For this review, take the finished solid that the model builds, in its own axes (mm). Face numbers are marked on the shaded views. Round coordinates to 2 decimals unless told otherwise and drop trailing zeros. Order: outer loops, then holes, each group sorted by start corner. A loop starts at its lowest first (then second) coordinate and runs counter-clockwise, first axis right, second up. Notation, with made-up numbers: M -10,-11 L 6,-11 A11 cw 6,7 Z; hole C -3,2.25 d5. An arc over 180 degrees is marked long. Put each result on its own line as item: value.
from build123d import *

# Parameters (mm, degrees)
SKETCH1_R           = 1.7859375
SKETCH1_R_2         = 12.7
BOSS_EXTRUDE1_DEPTH = 3.175
SKETCH2_W           = 6.35
SKETCH2_H           = 38.1
BOSS_EXTRUDE2_DEPTH = 17.7165
SKETCH3_W           = 50.8
SKETCH3_H           = 38.1
SKETCH3_R           = 4.7625
BOSS_EXTRUDE3_DEPTH = 3.175
SKETCH4_W           = 6.35
SKETCH4_H           = 38.1
BOSS_EXTRUDE4_DEPTH = 6.35
FILLET1_R           = 2.54
CUT_EXTRUDE2_REACH  = 94.617
SKETCH6_R           = 1.7859375


with BuildPart() as part:
    # Sketch1 → Boss-Extrude1 (new body)
    with BuildSketch(Plane.XY):
        Polygon((25.4, -19.05), (25.4, 49.157882323), (61.857882323, 49.157882323), (61.857882323, 61.857882323), (19.05, 61.857882323), (-19.05, 61.857882323), (-61.857882323, 61.857882323), (-61.857882323, 49.157882323), (-25.4, 49.157882323), (-25.4, -19.05), (-25.4, -49.157882323), (-61.857882323, -49.157882323), (-61.857882323, -61.857882323), (-19.05, -61.857882323), (19.05, -61.857882323), (61.857882323, -61.857882323), (61.857882323, -49.157882323), (25.4, -49.157882323), align=None)
        with Locations((-55.507882323, -55.507882323)):
            Circle(SKETCH1_R, mode=Mode.SUBTRACT)
        with Locations((55.507882323, -55.507882323)):
            Circle(SKETCH1_R, mode=Mode.SUBTRACT)
        Circle(SKETCH1_R_2, mode=Mode.SUBTRACT)
        with Locations((-55.507882323, 55.507882323)):
            Circle(SKETCH1_R, mode=Mode.SUBTRACT)
        with Locations((55.507882323, 55.507882323)):
            Circle(SKETCH1_R, mode=Mode.SUBTRACT)
    extrude(amount=BOSS_EXTRUDE1_DEPTH)

    # Sketch2 → Boss-Extrude2 (add)
    with BuildSketch(Plane.XY.offset(3.175)):
        with Locations((22.225, 0)):
            Rectangle(SKETCH2_W, SKETCH2_H)
        with Locations((-22.225, 0)):
            Rectangle(SKETCH2_W, SKETCH2_H)
    extrude(amount=BOSS_EXTRUDE2_DEPTH)

    # Sketch3 → Boss-Extrude3 (add)
    with BuildSketch(Plane.XY.offset(20.8915)):
        Rectangle(SKETCH3_W, SKETCH3_H)
        Circle(SKETCH3_R, mode=Mode.SUBTRACT)
    extrude(amount=BOSS_EXTRUDE3_DEPTH)

    # Sketch4 → Boss-Extrude4 (add)
    with BuildSketch(Plane.XY.offset(24.0665)):
        with Locations((11.0236, 0)):
            Rectangle(SKETCH4_W, SKETCH4_H)
        with Locations((-11.0236, 0)):
            Rectangle(SKETCH4_W, SKETCH4_H)
    extrude(amount=BOSS_EXTRUDE4_DEPTH)

    # Fillet1
    fillet1_edges = [part.edges().sort_by_distance(p)[0] for p in [
        (61.857882323, -49.157882323, 1.5875),
        (61.857882323, -61.857882323, 1.5875),
        (-61.857882323, -61.857882323, 1.5875),
        (-61.857882323, -49.157882323, 1.5875),
        (-25.4, -49.157882323, 1.5875),
        (-25.4, 49.157882323, 1.5875),
        (-61.857882323, 49.157882323, 1.5875),
        (-61.857882323, 61.857882323, 1.5875),
        (61.857882323, 61.857882323, 1.5875),
        (61.857882323, 49.157882323, 1.5875),
        (25.4, 49.157882323, 1.5875),
        (25.4, -49.157882323, 1.5875),
    ]]
    fillet(fillet1_edges, radius=FILLET1_R)

    # Sketch6 → Cut-Extrude2 (cut, up to next)
    with BuildSketch(Plane(origin=(0, 0, 0), x_dir=(-1, 0, 0), z_dir=(0, 0, -1)), mode=Mode.PRIVATE) as cut_extrude2_sk1:
        with Locations((-22.225, -12.7)):
            Circle(SKETCH6_R)
    cut_extrude2_tool1 = extrude(cut_extrude2_sk1.sketch, amount=-CUT_EXTRUDE2_REACH, mode=Mode.PRIVATE) & part.part
    # Sketch6 → Cut-Extrude2 (cut, up to next)
    with BuildSketch(Plane(origin=(0, 0, 0), x_dir=(-1, 0, 0), z_dir=(0, 0, -1)), mode=Mode.PRIVATE) as cut_extrude2_sk2:
        with Locations((-22.225, 12.7)):
            Circle(SKETCH6_R)
    cut_extrude2_tool2 = extrude(cut_extrude2_sk2.sketch, amount=-CUT_EXTRUDE2_REACH, mode=Mode.PRIVATE) & part.part
    # Sketch6 → Cut-Extrude2 (cut, up to next)
    with BuildSketch(Plane(origin=(0, 0, 0), x_dir=(-1, 0, 0), z_dir=(0, 0, -1)), mode=Mode.PRIVATE) as cut_extrude2_sk3:
        with Locations((22.225, 12.7)):
            Circle(SKETCH6_R)
    cut_extrude2_tool3 = extrude(cut_extrude2_sk3.sketch, amount=-CUT_EXTRUDE2_REACH, mode=Mode.PRIVATE) & part.part
    # Sketch6 → Cut-Extrude2 (cut, up to next)
    with BuildSketch(Plane(origin=(0, 0, 0), x_dir=(-1, 0, 0), z_dir=(0, 0, -1)), mode=Mode.PRIVATE) as cut_extrude2_sk4:
        with Locations((22.225, -12.7)):
            Circle(SKETCH6_R)
    cut_extrude2_tool4 = extrude(cut_extrude2_sk4.sketch, amount=-CUT_EXTRUDE2_REACH, mode=Mode.PRIVATE) & part.part
    add(cut_extrude2_tool1.solids().sort_by_distance((22.225, -12.7, 0))[0], mode=Mode.SUBTRACT)
    add(cut_extrude2_tool2.solids().sort_by_distance((22.225, 12.7, 0))[0], mode=Mode.SUBTRACT)
    add(cut_extrude2_tool3.solids().sort_by_distance((-22.225, 12.7, 0))[0], mode=Mode.SUBTRACT)
    add(cut_extrude2_tool4.solids().sort_by_distance((-22.225, -12.7, 0))[0], mode=Mode.SUBTRACT)


solid = part.part
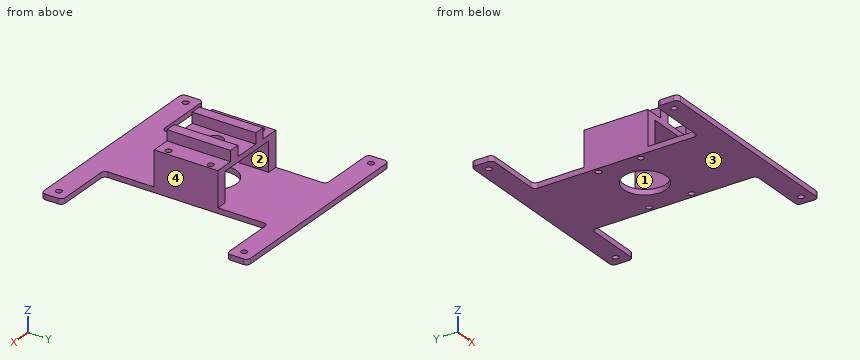
(1) Draft analysis for pull direction Z (two halves, no side actions). For the marked faces 1, 2, 3 and 4, state which applies: released by +Z, released by -Z, zero draft, split by the parting line, or undercut.
A:
face 1: undercut
face 2: undercut
face 3: released by -Z
face 4: zero draft
(2) To check wall thickness, follow L1, parallel to X at y = -8, z = 16; L2, parallel to Y at x = -6.5, z = 2; L3, parallel to Z at x = 13.5, y = -13 (1 decimal). State the ranges of each line that lie inside material, in increasing order.
A:
L1: x = -25.4 to -19.05, 19.05 to 25.4
L2: y = -61.86 to -10.91, 10.91 to 61.86
L3: z = 0 to 3.2, 20.9 to 30.4
(3) Insertion check: pin 1 Ø1.9 at (y, z) = (-6.5, 26.5) entering from -X; pin 2 Ø5.5 at (x, y) = (-17, -4.5) entering from +Z; pin 3 Ø5.5 at (x, y) = (-55.51, 55.51) entering from +Z (3 decimals); pin 4 Ø3 at (x, y) = (22.225, 12.7) entering from -Z. Each pin has a flat end and moves straight along its axis. Give the tip position at first contact, or say it passes through.
A:
pin 1: stops at x = -14.2
pin 2: stops at z = 24.07
pin 3: stops at z = 3.175
pin 4: passes through
(4) Add section D-D on z = 25.5. Give the boundary of the cut face in (x, y).
A:
outline: M -14.2,-19.05 L -7.85,-19.05 L -7.85,19.05 L -14.2,19.05 Z; M 7.85,-19.05 L 14.2,-19.05 L 14.2,19.05 L 7.85,19.05 Z
(5) Add section C-C on x = 40. Give the boundary of the cut face in (y, z) (3 decimals), then the cut area to 3 significant figures.
A:
outline: M -61.858,0 L -49.158,0 L -49.158,3.175 L -61.858,3.175 Z; M 49.158,0 L 61.858,0 L 61.858,3.175 L 49.158,3.175 Z
area: 80.6 mm2
(6) Add section A-A on z = 19. Give the boundary of the cut face in (x, y) (3 decimals).
A:
outline: M -25.4,-19.05 L -19.05,-19.05 L -19.05,19.05 L -25.4,19.05 Z; M 19.05,-19.05 L 25.4,-19.05 L 25.4,19.05 L 19.05,19.05 Z; hole C -22.225,-12.7 d3.572; hole C -22.225,12.7 d3.572; hole C 22.225,-12.7 d3.572; hole C 22.225,12.7 d3.572
